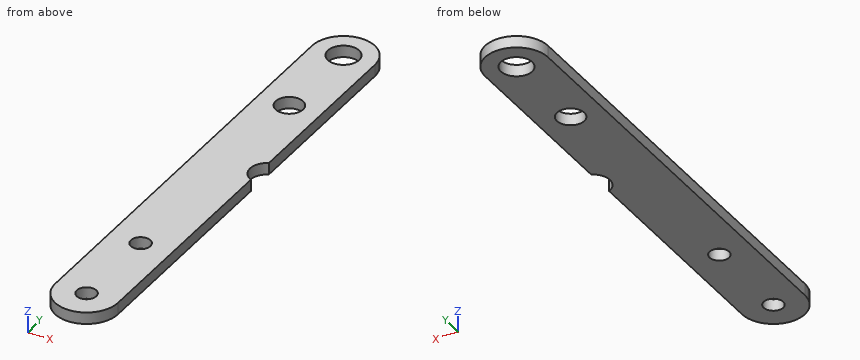
```python
from build123d import *

# Parameters (mm, degrees)
F1_R     = 7.9375
F1_R_2   = 11.1125
F1_R_3   = 12.7
F2_DEPTH = 9.525


with BuildPart() as f2:
    # F1 (on Top) → F2 (new body)
    with BuildSketch(Plane.XY):
        with BuildLine():
            ThreePointArc((25.399975, 180.975), (-1.3e-05, 206.374987), (-25.4, 180.975))
            Line((-25.4, 180.975), (-25.4, -180.975))
            ThreePointArc((-25.4, -180.975), (-1.3e-05, -206.374987), (25.399975, -180.975))
            Line((25.399975, -180.975), (25.399975, 6.35))
            ThreePointArc((25.399975, 6.35), (17.474131, 19.05), (25.399975, 31.75))
            Line((25.399975, 31.75), (25.399975, 180.975))
        make_face()
        with Locations((-2.5e-05, -180.975)):
            Circle(F1_R, mode=Mode.SUBTRACT)
        with Locations((-2.5e-05, -104.775)):
            Circle(F1_R, mode=Mode.SUBTRACT)
        with Locations((-2.5e-05, 104.775)):
            Circle(F1_R_2, mode=Mode.SUBTRACT)
        with Locations((-2.5e-05, 180.975)):
            Circle(F1_R_3, mode=Mode.SUBTRACT)
    extrude(amount=F2_DEPTH)


solid = f2.part
```
The model under review builds one solid part; all positions refer to its coordinate system, in mm. Round coordinates to 2 decimals unless told otherwise and drop trailing zeros. Write each loop counter-clockwise with the first axis right and the second up, starting at its lowest first coordinate (ties: lowest second). Pieces come first, ordered by that corner, then holes.
(1) We need section C-C on y = 25. Give the boundary of the cut face in (x, z) (3 decimals), and give its area (3 significant figures).
(2) We need section B-B on z = 2.5. Give the number of separate pieces and of enclosed holes in the cut face, and give its area (3 significant figures).
(3) Insertion check: pin 1 (3 mm diameter, centred on x = -8.5, z = 7.5, fed in from -Y). The pin has a flat end and moves straight along its axis. Give the tip position at first contact, or say it passes through.
(4) We need section A-A on x = 3. Give the boundary of the cut face in (y, z) (3 decimals), and give its area (3 significant figures).
(5) Wall thickness on L1, parallel to Y at x = 3.5, z = 6.5; L2, parallel to X at y = 102, z = 1.5; L3, parallel to Y at x = -11.5, z = 4: over which ranges is each line inside the solid? List them lowest first.
Findings below:
1. outline: (-25.4, 0) - (18.787, 0) - (18.787, 9.525) - (-25.4, 9.525) - close
1. area: 421 mm2
2. separate pieces: 1
2. enclosed holes: 4
2. area: 19,000 mm2
3. pin 1: stops at y = -205.39
4. outline: (-206.197, 0) - (-188.324, 0) - (-188.324, 9.525) - (-206.197, 9.525) - close; (-173.626, 0) - (-112.124, 0) - (-112.124, 9.525) - (-173.626, 9.525) - close; (-97.426, 0) - (94.075, 0) - (94.075, 9.525) - (-97.426, 9.525) - close; (115.475, 0) - (168.634, 0) - (168.634, 9.525) - (115.475, 9.525) - close; (193.316, 0) - (206.197, 0) - (206.197, 9.525) - (193.316, 9.525) - close
4. area: 3,210 mm2
5. L1: y = -206.13 to -188.1, -173.85 to -111.9, -97.65 to 94.23, 115.32 to 168.77, 193.18 to 206.13
5. L2: x = -25.4 to -10.76, 10.76 to 25.4
5. L3: y = -203.62 to 175.59, 186.36 to 203.62
